```python
from build123d import *

# Parameters (mm, degrees)
F0_W     = 30
F0_H     = 30
F1_DEPTH = 42
F2_R     = 6.75
F3_DEPTH = 12
F6_W     = 3
F6_H     = 3
F7_DEPTH = 1
F8_R     = 0.75
F9_DEPTH = 8.2927961675


with BuildPart() as f1:
    # F0 (on Top) → F1 (new body)
    with BuildSketch(Plane.XY):
        Rectangle(F0_W, F0_H)
    extrude(amount=F1_DEPTH)

    # F2 (on Top) → F3 (cut)
    with BuildSketch(Plane.XY):
        Circle(F2_R)
    extrude(amount=F3_DEPTH, mode=Mode.SUBTRACT)

    # F4 (on Front) → F5 (revolve, cut)
    with BuildSketch(Plane.XZ):
        Polygon((0, 9.4530368224), (0, 0), (10, 0), align=None)
    revolve(axis=Axis((0, 0, 4.7265184112), (0, 0, -1)), mode=Mode.SUBTRACT)

    # F6 (on face) → F7 (join)
    with BuildSketch(Plane.XY.offset(42)):
        with Locations((-13.5, 13.5)):
            Rectangle(F6_W, F6_H)
        with Locations((13.5, 13.5)):
            Rectangle(F6_W, F6_H)
        with Locations((13.5, -13.5)):
            Rectangle(F6_W, F6_H)
        with Locations((-13.5, -13.5)):
            Rectangle(F6_W, F6_H)
    extrude(amount=F7_DEPTH)

    # F8 (on face) → F9 (cut, through all)
    with BuildSketch(Plane.YZ.offset(15)):
        with Locations((0, 11)):
            Circle(F8_R)
    extrude(amount=-F9_DEPTH, mode=Mode.SUBTRACT)


solid = f1.part
```
The listing builds one solid part. Answer for the finished solid, in the listing's coordinates (mm). A direction names the side the tool comes from. Coordinates: 2 decimals unless noted, no trailing zeros. Loops run counter-clockwise (first coordinate to the right, second up) from the corner with the lowest first, then second, coordinate; pieces in that order, holes last. Notation, with made-up numbers: (77.5, 44.5) -> (118.5, 44.5) arc R25 cw to (118.5, 65.5) -> close; hole circle Ø3 at (-35.5, 61). An arc over 180 degrees is marked (long way). Return JSON: item names as keys, results as strings. Group by question number.
(1) Find the intervals of material crossed by probe 1 along Y at (x, z) = (0, 5); probe 2 along Y at (x, z) = (9, 11), in increasing order. Write a range as from..to.
(2) A cutting plane is placed at C-C on x = 0. Write down the section's boundary in (y, z).
(3) A cutting plane is placed at D-D on y = 11.5. Write down the section's boundary in (x, z), and give its area (3 significant figures).
(4) A cutting plane is placed at A-A on y = 0. Write down the section's boundary in (x, z).
(5) Given pin 1 Ø7 at (x, y) = (2, 2.5) entering from -Z; pin 2 Ø9 at (x, y) = (-3.5, 1.5) entering from +Z; pin 3 Ø6 at (x, y) = (-3.5, 3) entering from -Z; pin 4 Ø1.7 at (y, z) = (0, 11) entering from +X, each flat-ended and moving along its own axis, determine where each tip first touches the part or whether it passes through.
(6) Determine the mould class of faces 1 (the flat face through (-12, 13.5, 42.5)), 2 (the flat face through (-0.2, 10.2, 0)), 3 (the cylindrical face through (10.912, -0.098, 11.744)) for opening direction Z: released by +Z, released by -Z, zero draft, split by the parting line, or undercut.
(7) A cutting plane is placed at B-B on z = 11. Write down the section's boundary in (x, y), and give its area (3 significant figures).
(8) Which of the six approach directions +Z, -Z, +X, -X, +Y, -Y give full straight-line access (tool end or side, diameter ignored) to faces 4 (the flat face through (15, 0, 21)), 5 (the flat face through (-14, -13, 43)), 6 (the flat face through (12, -13.5, 42.5)), 7 (the flat face through (13.5, 12, 42.5)), 8 (the cylindrical face through (-1.46, -6.59, 7.47))?
The answers:
{
 "1": {"probe 1": "y = -15..-6.75, 6.75..15", "probe 2": "y = -15..-0.75, 0.75..15"},
 "2": {"outline": "(-15, 0) -> (-10, 0) -> (-6.75, 3.07) -> (-6.75, 12) -> (6.75, 12) -> (6.75, 3.07) -> (10, 0) -> (15, 0) -> (15, 42) -> (-15, 42) -> close"},
 "3": {"outline": "(-15, 0) -> (15, 0) -> (15, 42) -> (-15, 42) -> close", "area": "1,260 mm^2"},
 "4": {"outline": "(-15, 0) -> (-10, 0) -> (-6.75, 3.07) -> (-6.75, 12) -> (6.75, 12) -> (6.75, 11.75) -> (15, 11.75) -> (15, 42) -> (-15, 42) -> close; (6.75, 3.07) -> (10, 0) -> (15, 0) -> (15, 10.25) -> (6.75, 10.25) -> close"},
 "5": {"pin 1": "stops at z = 12", "pin 2": "stops at z = 42", "pin 3": "stops at z = 2.26", "pin 4": "stops at x = 15"},
 "6": {"face 1": "zero draft", "face 2": "released by -Z", "face 3": "undercut"},
 "7": {"outline": "(-15, -15) -> (15, -15) -> (15, -0.75) -> (6.71, -0.75) arc R6.75 cw (long way) to (6.71, 0.75) -> (15, 0.75) -> (15, 15) -> (-15, 15) -> close", "area": "744 mm^2"},
 "8": {"face 4": "+Z, -Z, +X, +Y, -Y", "face 5": "+Z, +X, -X, +Y, -Y", "face 6": "+Z, +Y, -Y", "face 7": "+Z, +X, -X", "face 8": "-Z"}
}
